Answer from the drawing. Dimensions are ordinates in mm from the lowest x, y and z of the part. A direction names the side the tool comes from. Round coordinates to 2 decimals unless told otherwise and drop trailing zeros. Loops run counter-clockwise (first coordinate to the right, second up) from the corner with the lowest first, then second, coordinate; pieces in that order, holes last. Notation, with made-up numbers: (83.25, 84) -> (130.25, 84) arc R13 ccw to (130.25, 94) -> close; hole circle Ø1 at (-8, 13). An arc over 180 degrees is marked (long way). One line per question, with ' | ' between items.
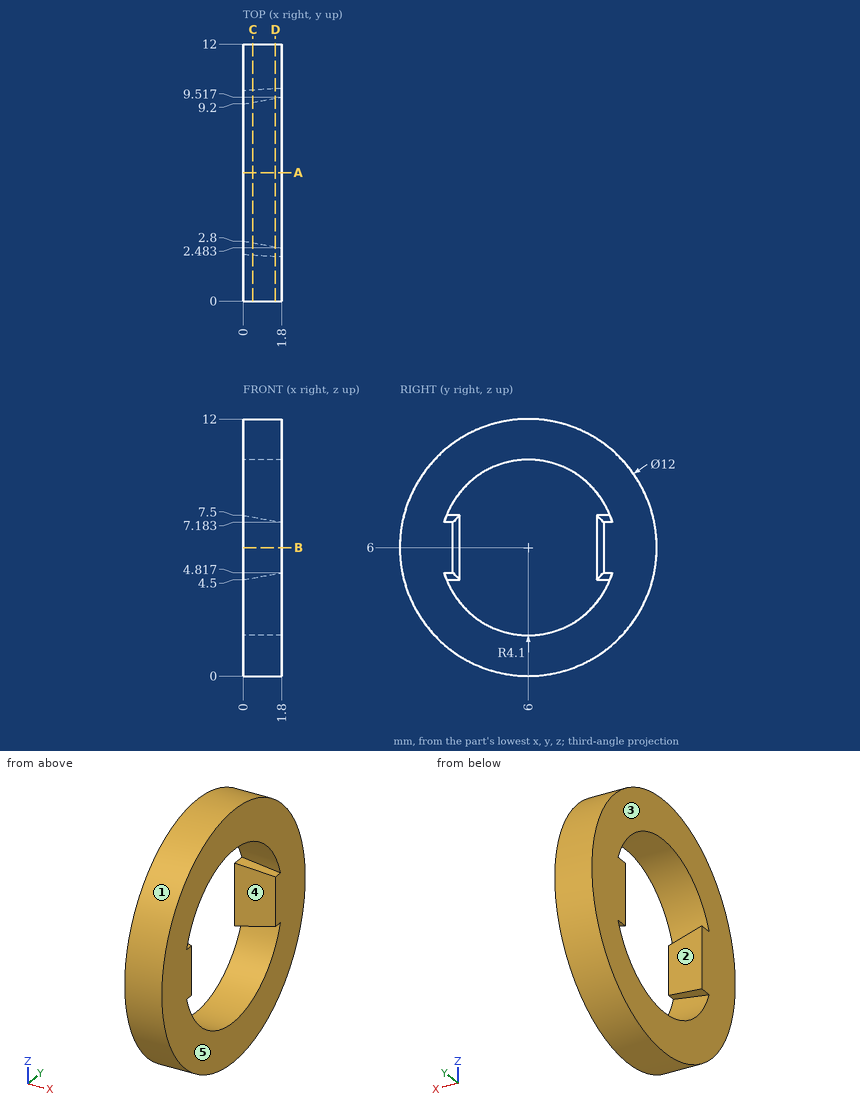
Q1. Find the intervals of material crossed by line 1 (Y direction, x = 0.45, z = 3.75); line 2 (Y direction, x = 0.7, z = 3) (1 decimal); line 3 (Z direction, x = 1, y = 4), in increasing order. Write a range as from..to.
Numbers:
line 1: 0.44..2.57, 9.43..11.56 | line 2: 0.8..3.2, 8.8..11.2 | line 3: 0.34..2.42, 9.58..11.66
Q2. Given pin 1 Ø1 at (x, z) = (1.5, 2) entering from -Y, flat-ended and moving along its own axis, determine where the tip first touches the part or whether it passes through.
Numbers:
pin 1: y = 1.13
Q3. A cutting plane is placed at A-A on y = 6. Give the vertices of the cut face in (x, z).
Numbers:
outline: (0, 0) -> (1.8, 0) -> (1.8, 1.9) -> (0, 1.9) -> close; (0, 10.1) -> (1.8, 10.1) -> (1.8, 12) -> (0, 12) -> close
Q4. A cutting plane is placed at D-D on x = 1.5. Give the vertices of the cut face in (y, z) (1 decimal).
Numbers:
outline: circle Ø12 at (6, 6); hole (2.1, 4.8) arc R4.1 ccw to (9.9, 4.8) -> (9.5, 4.8) -> (9.5, 7.2) -> (9.9, 7.2) arc R4.1 ccw to (2.1, 7.2) -> (2.5, 7.2) -> (2.5, 4.8) -> close
Q5. For a pull along Y with two mould halves and no side action, classify the marked faces 1, 2 and 3 as pulls with the +Y half, pulls with the -Y half, needs draft (parallel to the pull), parting line crosses it, or undercut.
Numbers:
face 1: parting line crosses it | face 2: undercut | face 3: needs draft
Q6. A cutting plane is placed at B-B on z = 6. Give the vertices of the cut face in (x, y).
Numbers:
outline: (0, 0) -> (1.8, 0) -> (1.8, 2.48) -> (0, 2.8) -> close; (0, 9.2) -> (1.8, 9.52) -> (1.8, 12) -> (0, 12) -> close
Q7. For the marked faces 4 and 5, determine the directions among +Z, -Z, +X, -X, +Y, -Y from which every point of the face is accessible in a straight line to the end or side of a thin tool.
Numbers:
face 4: +X | face 5: +Z, -Z, +X, +Y, -Y
Q8. A cutting plane is placed at C-C on x = 0.45. Give the vertices of the cut face in (y, z).
Numbers:
outline: circle Ø12 at (6, 6); hole (2.15, 4.58) arc R4.1 ccw to (9.85, 4.58) -> (9.28, 4.58) -> (9.28, 7.42) -> (9.85, 7.42) arc R4.1 ccw to (2.15, 7.42) -> (2.72, 7.42) -> (2.72, 4.58) -> close
